Geometry: final body of the model. Coordinates: model frame, mm. Coordinates: 2 decimals unless noted, no trailing zeros. Write each loop counter-clockwise with the first axis right and the second up, starting at its lowest first coordinate (ties: lowest second). Pieces come first, ordered by that corner, then holes. Notation, with made-up numbers: (60, -25) -> (101, -25) arc R28 cw to (101, -1) -> close; hole circle Ø9 at (-7, 56.5). An arc over 180 degrees is marked (long way). One line per item, written item: value.
```python
from build123d import *

# Parameters (mm, degrees)
CYLINDER001_R          = 3.2
CYLINDER001_DEPTH      = 10
CYLINDER001_ROLL_ANGLE = 90
CYLINDER_R             = 3.2
CYLINDER_DEPTH         = 10
CYLINDER_ROLL_ANGLE    = 90
PAD_DEPTH              = 50
CHAMFER_SIZE           = 2


with BuildPart() as cylinder001:
    # Cylinder001 → Cylinder001 (new body)
    with BuildSketch(Plane.XY):
        Circle(CYLINDER001_R)
    extrude(amount=CYLINDER001_DEPTH)


with BuildPart() as cylinder001_1:
    # Cylinder001 roll: moved
    add(cylinder001.part.rotate(Axis((0, 0, 0), (1, 0, 0)), CYLINDER001_ROLL_ANGLE))


with BuildPart() as cylinder001_2:
    # Cylinder001 placement: moved
    add(cylinder001_1.part.moved(Location((0, 2, -37.5))))


with BuildPart() as cylinder:
    # Cylinder → Cylinder (new body)
    with BuildSketch(Plane.XY):
        Circle(CYLINDER_R)
    extrude(amount=CYLINDER_DEPTH)


with BuildPart() as cylinder_1:
    # Cylinder roll: moved
    add(cylinder.part.rotate(Axis((0, 0, 0), (1, 0, 0)), CYLINDER_ROLL_ANGLE))


with BuildPart() as cylinder_2:
    # Cylinder placement: moved
    add(cylinder_1.part.moved(Location((0, 2, 37.5))))


with BuildPart() as chamfer_body:
    # Sketch001 → Pad (new body, symmetric)
    with BuildSketch(Plane.XY):
        with BuildLine():
            ThreePointArc((6, -5.97913), (0, -1.97913), (-6, -5.97913))
            Line((-5.5, 0), (-6, -5.97913))
            Line((-5.5, 0), (5.5, 0))
            Line((5.5, 0), (6, -5.97913))
        make_face()
    extrude(amount=PAD_DEPTH, both=True)

    # Cut: cut Cylinder
    add(cylinder_2.part, mode=Mode.SUBTRACT)

    # Cut002: cut Cylinder001
    add(cylinder001_2.part, mode=Mode.SUBTRACT)

    # Chamfer
    chamfer_edges = [chamfer_body.edges().sort_by_distance(p)[0] for p in [
        (6, -5.97913, 0),
        (-6, -5.97913, 0),
    ]]
    chamfer(chamfer_edges, length=CHAMFER_SIZE)


solid = chamfer_body.part
```
(1) First-contact query: pin 1 (4 mm diameter, centred on x = 0, z = 37.5, fed in from +Y). Flat tip, straight axial feed; report the tip coordinate or a pass-through.
Responses:
pin 1: passes through
(2) Section B-B (x = 0.25). Return the cut outline in (y, z), then the cut area to 3 significant figures.
Responses:
outline: (-1.98, -50) -> (0, -50) -> (0, -40.69) -> (-1.98, -40.69) -> close; (-1.98, -34.31) -> (0, -34.31) -> (0, 34.31) -> (-1.98, 34.31) -> close; (-1.98, 40.69) -> (0, 40.69) -> (0, 50) -> (-1.98, 50) -> close
area: 173 mm2
(3) Line query: line 1 (Z direction, x = 0, y = -1.8); line 2 (Z direction, x = 2.75, y = -0.65); line 3 (X direction, y = -3.25, z = -30). Output: solid intervals per line, ascending. Write a range as [from, to].
Responses:
line 1: z = [-50, -40.7], [-34.3, 34.3], [40.7, 50]
line 2: z = [-50, -39.14], [-35.86, 35.86], [39.14, 50]
line 3: x = [-5.77, -3.86], [3.86, 5.77]
(4) Section A-A (z = 37.5). Return the cut outline in (x, y), then the cut area to 3 significant figures.
Responses:
outline: (-5.83, -3.99) -> (-4.96, -4.27) arc R6.5 cw to (-3.2, -2.82) -> (-3.2, 0) -> (-5.5, 0) -> close; (3.2, -2.82) arc R6.5 cw to (4.96, -4.27) -> (5.83, -3.99) -> (5.5, 0) -> (3.2, 0) -> close
area: 18.1 mm2
(5) Pull-direction query (X, two-part tool) for faces 1 (the flat face through (5.664, -1.965, 0.7)), 2 (the flat face through (0, 0, 1)), 3 (the cylindrical face through (3.052, -1.077, -36.539)); classes: released by +X, released by -X, zero draft, split by the parting line, or undercut.
Responses:
face 1: released by +X
face 2: zero draft
face 3: undercut
